Autodesk Inventor part; units mm, degrees
ref_plane "YZ Plane" through (0, 0, 0) normal (1, 0, 0) x (0, 1, 0)
ref_plane "XZ Plane" through (0, 0, 0) normal (0, 1, 0) x (-1, 0, 0)
ref_plane "XY Plane" through (0, 0, 0) normal (0, 0, 1) x (1, 0, 0)
sketch "Sketch1" plane through (0, 0, 0) normal (1, 0, 0) x (0, 1, 0)
  point P0 (0, 0)
sketch "Sketch2" plane through (0, 0, 0) normal (1, 0, 0) x (0, 1, 0)
  line L0 (500, 175) -> (0, 175)
  line L1 (0, 175) -> (0, -175)
  line L2 (0, -175) -> (500, -175)
  line L3 (500, -175) -> (500, 175)
  point P0 (0, 0)
  dimension "d0" = 500
  dimension "d1" = 350
  dimension "d2" = 175
  dimension "d3" = 500
extrude "Extrusion1" add sketch "Sketch2" along normal blind 300
sketch "Sketch3" plane through (300, 0, 0) normal (1, 0, 0) x (0, 0, -1)
  circle A0 centre (0, 350) radius 100
  point P0 (0, 0)
  dimension "d6" = 200
  dimension "d7" = 350
extrude "Extrusion2" cut sketch "Sketch3" against normal blind 10
sketch "Sketch6" plane through (290, 350, 0) normal (1, 0, 0) x (0, 0, -1)
  line L0 (-0.0604, -0.1466) -> (-75.0604, -0.1466)
  line L1 (-75.0604, -0.1466) -> (-0.0604, -0.1466)
  line L2 (-0.0604, -0.1466) -> (-73.5885, 14.6388)
  line L3 (-0.0604, -0.1466) -> (-67.2185, 33.4039)
  line L4 (-0.0604, -0.1466) -> (-58.5037, 46.9726)
  line L5 (-0.0604, -0.1466) -> (-45.1893, 59.847)
  line L6 (-0.0604, -0.1466) -> (-31.7085, 67.9287)
  line L7 (-0.0604, -0.1466) -> (-13.5499, 73.7038)
  line L8 (-0.0604, -0.1466) -> (11.8236, 73.9791)
  arc A0 (-73.5885, 14.6388) -> (-75.0604, -0.1466) centre (-37.9126, 3.6215) ccw
  arc A1 (-58.5037, 46.9726) -> (-67.2185, 33.4039) centre (-31.8389, 20.2637) ccw
  arc A2 (-31.7085, 67.9287) -> (-45.1893, 59.847) centre (-16.7307, 27.6606) ccw
  arc A3 (11.8236, 73.9791) -> (-13.5499, 73.7038) centre (-0.4454, 35.3353) ccw
  line L9 (-0.0604, -0.1466) -> (64.6218, 36.8812)
  line L10 (-0.0604, -0.1466) -> (51.5848, 53.6216)
  line L11 (-0.0604, -0.1466) -> (40.3954, 64.3692)
  line L12 (-0.0604, -0.1466) -> (23.8014, 71.9871)
  arc A4 (40.3954, 64.3692) -> (23.8014, 71.9871) centre (16.5753, 34.3639) ccw
  arc A5 (64.6218, 36.8812) -> (51.5848, 53.6216) centre (33.1363, 25.8077) ccw
  arc A6 (74.9396, -0.1466) -> (73.8878, 16.2903) centre (21.7524, 4.7019) ccw
  line L13 (73.8878, 16.2903) -> (-0.0604, -0.1466)
  line L14 (74.9396, -0.1466) -> (-0.0604, -0.1466)
  point P0 (0, -350)
  dimension "d18" = 75
  dimension "d20" = 11.37
  dimension "d21" = 75
extrude "Extrusion3" cut sketch "Sketch6" against normal blind 3
sketch "Sketch7" plane through (300, 0, 0) normal (1, 0, 0) x (0, 0, -1)
  circle A0 centre (0, 100) radius 10
  point P0 (0, 0)
  dimension "d24" = 100
  dimension "d25" = 20
extrude "Extrusion4" cut sketch "Sketch7" against normal blind 150
equation "\"d21\" = d18"
properties part number "holder"
Could you check a few things on this model? Use its own coordinates, in mm. A direction names the side the tool comes from. Give positions to 0.01 mm unless a question says otherwise; leave off trailing zeros. Order: outer loops, then holes, each group sorted by start corner. A loop starts at its lowest first (then second) coordinate and runs counter-clockwise, first axis right, second up. Notation, with made-up numbers: M 44.25,54 L 51.25,54 A31 ccw 51.25,85 Z; hole C 86.5,52.25 d5. An arc over 180 degrees is marked long. One line per question, with ' | ' between items.
1. I want a section at A-A (y = 100). List the corners of the cut face in (x, z) for me, and give its area (3 significant figures).
Results:
outline: M 0,-175 L 300,-175 L 300,-10 L 150,-10 L 150,10 L 300,10 L 300,175 L 0,175 Z | area: 102,000 mm²
2. I want a section at B-B (y = 297.5). List the corners of the cut face in (x, z) for me, and give its area (3 significant figures).
Results:
outline: M 0,-175 L 300,-175 L 300,-85.11 L 290,-85.11 L 290,85.11 L 300,85.11 L 300,175 L 0,175 Z | area: 103,000 mm²
3. I'm going to push flat-ended pins straight in: pin 1 (5 mm diameter, centred on y = 359, z = -50.5, fed in from +X); pin 2 (6 mm diameter, centred on y = 101, z = 3.5, fed in from +X). Where does each tip first touch, or does it pass through?
Results:
pin 1: x = 290 | pin 2: x = 150
4. We'd pull the mould along Z, two halves only. Please class faces 3 (the face through (288.521, 357.143, 36.31)), 4 (the face through (148, 253, 175)), 5 (the face through (148, 0, 2)): +Z half, -Z half, draft (parallel to the pull), parting line (faces both ways), or undercut.
Results:
face 3: undercut | face 4: +Z half | face 5: draft
5. For faces 1 (the face through (0, 247, 2)), 2 (the face through (150, 100, 0)), which set-ups out of +Z, -Z, +X, -X, +Y, -Y let a thin tool reach every point of the face, with its end or its side?
Results:
face 1: +Z, -Z, -X, +Y, -Y | face 2: +X
6. If I drill on line 1 (Y direction, x = 294, z = 0); line 2 (Y direction, x = 247, z = 0); line 3 (X direction, y = 275.5, z = -55), over which ranges is the centre line in solid material (lowest first)?
Results:
line 1: 0 to 90, 110 to 250, 450 to 500 | line 2: 0 to 90, 110 to 500 | line 3: 0 to 290
